Read the model definition and answer for the solid it produces. Units are mm, in the model's axes. A direction names the side the tool comes from. Coordinates: 2 decimals unless noted, no trailing zeros. Loops run counter-clockwise (first coordinate to the right, second up) from the corner with the lowest first, then second, coordinate; pieces in that order, holes last.
Q1. Section C-C (y = 0.3) is taken. Count the separate pieces of the cut face and the enclosed holes in it, then the cut area to 3 significant figures.
Q2. Flat-ended cylindrical pins translate along their axes: P1, Ø0.8, axis at y = 1, z = 2.5, coming from the +X side; P2, Ø0.5, axis at x = 29.5, y = 1, coming from the +Z side; P3, Ø0.8, axis at y = 0.5, z = -3.5, coming from the -X side. Find the tip coordinate at first contact, or state that the pin passes through.
Q3. The mould has two halves that part along X. Classify faces 6 (the face through (7.913, 0.838, 11.535)), 7 (the face through (36.823, 0.838, -16.446)), 8 (the face through (27.461, 0.838, -15.786)), 9 (the face through (1, 1.7, 0)): pulls with the +X half, pulls with the -X half, needs draft (parallel to the pull), parting line crosses it, or undercut.
Q4. Straight lines are drawn through the part: line 1 (X direction, y = 0.6, z = 15) (3 decimals); line 2 (X direction, y = 1.25, z = -18); line 3 (Z direction, x = 33, y = 0.3). For each, find the intervals that lie inside material, in ascending order.
Q5. Which of the six approach directions +Z, -Z, +X, -X, +Y, -Y give full straight-line access (tool end or side, diameter ignored) to faces 1 (the face through (37, 1, 0)), 2 (the face through (-32.99, 0.84, 8.85)), 3 (the face through (-19.84, 0.84, -8.9)), 4 (the face through (27.213, 0.838, -21.413)), 5 (the face through (-30, 1, 21))?
Q6. Section B-B (z = 15) is taken. Give the vertices of the cut face in (x, y) (3 decimals).
Q7. Section A-A (z = 0) is taken. Give the vertices of the cut face in (x, y) (3 decimals), then the cut area to 3 significant figures.
from build123d import *

# Parameters (mm, degrees)
SKETCH1_R           = 6
SKETCH1_R_2         = 3.625
BOSS_EXTRUDE1_DEPTH = 1.7
CUT_EXTRUDE1_REACH  = 46.687
SKETCH2_W           = 13.125
SKETCH2_H           = 18.5
FILLET1_R           = 3
FILLET2_R           = 2


with BuildPart() as part:
    # Sketch1 → Boss-Extrude1 (new body)
    # profile 1 of 7: a face of its own
    with BuildSketch(Plane(origin=(0, 0, 0), x_dir=(1, 0, 0), z_dir=(0, 1, 0))):
        with BuildLine():
            Line((24.690598923, 25), (-24.690598923, 25))
            Line((-24.690598923, 25), (-27, 21))
            Line((-27, 21), (-31, 21))
            ThreePointArc((-31, 21), (-26.757359313, 19.242640687), (-25, 15))
            ThreePointArc((-25, 15), (-27.325765386, 10.25658351), (-32.5, 9.190524981))
            Line((-32.5, 9.190524981), (-32.5, 5.809475019))
            ThreePointArc((-32.5, 5.809475019), (-27.325765386, 4.74341649), (-25, 0))
            ThreePointArc((-25, 0), (-27.325765386, -4.74341649), (-32.5, -5.809475019))
            Line((-32.5, -5.809475019), (-32.5, -9.190524981))
            ThreePointArc((-32.5, -9.190524981), (-27.325765386, -10.25658351), (-25, -15))
            ThreePointArc((-25, -15), (-26.757359313, -19.242640687), (-31, -21))
            Line((-31, -21), (-27, -21))
            Line((-27, -21), (-24.690598923, -25))
            Line((-24.690598923, -25), (24.690598923, -25))
            Line((24.690598923, -25), (27, -21))
            Line((27, -21), (31, -21))
            ThreePointArc((31, -21), (25.047821822, -14.243974245), (32.5, -9.190524981))
            Line((32.5, -9.190524981), (32.5, -5.809475019))
            ThreePointArc((32.5, -5.809475019), (25, 0), (32.5, 5.809475019))
            Line((32.5, 5.809475019), (32.5, 9.190524981))
            ThreePointArc((32.5, 9.190524981), (25.047821822, 14.243974245), (31, 21))
            Line((31, 21), (27, 21))
            Line((27, 21), (24.690598923, 25))
        make_face()
    # profile 2 of 7: a face of its own
    with BuildSketch(Plane(origin=(0, 0, 0), x_dir=(1, 0, 0), z_dir=(0, 1, 0))):
        with Locations((-31, 15)):
            Circle(SKETCH1_R)
        with Locations(Location((-31, 15, 0), (0, 0, 270))):
            Circle(SKETCH1_R_2, mode=Mode.SUBTRACT)
    # profile 3 of 7: a face of its own
    with BuildSketch(Plane(origin=(0, 0, 0), x_dir=(1, 0, 0), z_dir=(0, 1, 0))):
        with Locations((-31, 0)):
            Circle(SKETCH1_R)
        with Locations(Location((-31, 0, 0), (0, 0, 270))):
            Circle(SKETCH1_R_2, mode=Mode.SUBTRACT)
    # profile 4 of 7: a face of its own
    with BuildSketch(Plane(origin=(0, 0, 0), x_dir=(1, 0, 0), z_dir=(0, 1, 0))):
        with Locations((-31, -15)):
            Circle(SKETCH1_R)
        with Locations(Location((-31, -15, 0), (0, 0, 270))):
            Circle(SKETCH1_R_2, mode=Mode.SUBTRACT)
    # profile 5 of 7: a face of its own
    with BuildSketch(Plane(origin=(0, 0, 0), x_dir=(1, 0, 0), z_dir=(0, 1, 0))):
        with Locations((31, -15)):
            Circle(SKETCH1_R)
        with Locations(Location((31, -15, 0), (0, 0, 270))):
            Circle(SKETCH1_R_2, mode=Mode.SUBTRACT)
    # profile 6 of 7: a face of its own
    with BuildSketch(Plane(origin=(0, 0, 0), x_dir=(1, 0, 0), z_dir=(0, 1, 0))):
        with Locations((31, 0)):
            Circle(SKETCH1_R)
        with Locations(Location((31, 0, 0), (0, 0, 270))):
            Circle(SKETCH1_R_2, mode=Mode.SUBTRACT)
    # profile 7 of 7: a face of its own
    with BuildSketch(Plane(origin=(0, 0, 0), x_dir=(1, 0, 0), z_dir=(0, 1, 0))):
        with Locations((31, 15)):
            Circle(SKETCH1_R)
        with Locations(Location((31, 15, 0), (0, 0, 270))):
            Circle(SKETCH1_R_2, mode=Mode.SUBTRACT)
    extrude(amount=BOSS_EXTRUDE1_DEPTH)

    # Sketch2 → Cut-Extrude1 (cut, up to next)
    with BuildSketch(Plane(origin=(0, 1.7, 0), x_dir=(1, 0, 0), z_dir=(0, 1, 0)), mode=Mode.PRIVATE) as cut_extrude1_sk1:
        with Locations((-13.6875, 0)):
            Rectangle(SKETCH2_W, SKETCH2_H)
    cut_extrude1_tool1 = extrude(cut_extrude1_sk1.sketch, amount=-CUT_EXTRUDE1_REACH, mode=Mode.PRIVATE) & part.part
    # Sketch2 → Cut-Extrude1 (cut, up to next)
    with BuildSketch(Plane(origin=(0, 1.7, 0), x_dir=(1, 0, 0), z_dir=(0, 1, 0)), mode=Mode.PRIVATE) as cut_extrude1_sk2:
        Polygon((-7.125, 9.25), (-7.125, 12.5), (-20.25, 9.25), align=None)
    cut_extrude1_tool2 = extrude(cut_extrude1_sk2.sketch, amount=-CUT_EXTRUDE1_REACH, mode=Mode.PRIVATE) & part.part
    # Sketch2 → Cut-Extrude1 (cut, up to next)
    with BuildSketch(Plane(origin=(0, 1.7, 0), x_dir=(1, 0, 0), z_dir=(0, 1, 0)), mode=Mode.PRIVATE) as cut_extrude1_sk3:
        Polygon((-7.125, -12.5), (-7.125, -9.25), (-20.25, -9.25), align=None)
    cut_extrude1_tool3 = extrude(cut_extrude1_sk3.sketch, amount=-CUT_EXTRUDE1_REACH, mode=Mode.PRIVATE) & part.part
    # Sketch2 → Cut-Extrude1 (cut, up to next)
    with BuildSketch(Plane(origin=(0, 1.7, 0), x_dir=(1, 0, 0), z_dir=(0, 1, 0)), mode=Mode.PRIVATE) as cut_extrude1_sk4:
        Polygon((7.125, -12.5), (20.25, -9.25), (7.125, -9.25), align=None)
    cut_extrude1_tool4 = extrude(cut_extrude1_sk4.sketch, amount=-CUT_EXTRUDE1_REACH, mode=Mode.PRIVATE) & part.part
    # Sketch2 → Cut-Extrude1 (cut, up to next)
    with BuildSketch(Plane(origin=(0, 1.7, 0), x_dir=(1, 0, 0), z_dir=(0, 1, 0)), mode=Mode.PRIVATE) as cut_extrude1_sk5:
        with Locations((13.6875, 0)):
            Rectangle(SKETCH2_W, SKETCH2_H)
    cut_extrude1_tool5 = extrude(cut_extrude1_sk5.sketch, amount=-CUT_EXTRUDE1_REACH, mode=Mode.PRIVATE) & part.part
    # Sketch2 → Cut-Extrude1 (cut, up to next)
    with BuildSketch(Plane(origin=(0, 1.7, 0), x_dir=(1, 0, 0), z_dir=(0, 1, 0)), mode=Mode.PRIVATE) as cut_extrude1_sk6:
        Polygon((20.25, 9.25), (7.125, 12.5), (7.125, 9.25), align=None)
    cut_extrude1_tool6 = extrude(cut_extrude1_sk6.sketch, amount=-CUT_EXTRUDE1_REACH, mode=Mode.PRIVATE) & part.part
    add(cut_extrude1_tool1.solids().sort_by_distance((-13.6875, 1.7, 0))[0], mode=Mode.SUBTRACT)
    add(cut_extrude1_tool2.solids().sort_by_distance((-11.5, 1.7, -10.333333))[0], mode=Mode.SUBTRACT)
    add(cut_extrude1_tool3.solids().sort_by_distance((-11.5, 1.7, 10.333333))[0], mode=Mode.SUBTRACT)
    add(cut_extrude1_tool4.solids().sort_by_distance((11.5, 1.7, 10.333333))[0], mode=Mode.SUBTRACT)
    add(cut_extrude1_tool5.solids().sort_by_distance((13.6875, 1.7, 0))[0], mode=Mode.SUBTRACT)
    add(cut_extrude1_tool6.solids().sort_by_distance((11.5, 1.7, -10.333333))[0], mode=Mode.SUBTRACT)

    # Fillet1
    # the kernel refuses this fillet: 3 mm, written as the material it adds along each edge
    with BuildSketch(Plane(origin=(32.5, 0, 9.190524981), x_dir=(0, 0, -1), z_dir=(0, 1, 0)), Plane(origin=(32.5, 0, -5.809475019), x_dir=(0, 0, -1), z_dir=(0, 1, 0))) as fillet1_piece_1:
        with BuildLine():
            CenterArc((1.984753615, -3), FILLET1_R, 90, 60)
            ThreePointArc((-0.613322597, -1.5), (-0.255786259, -0.770801874), (0, 0))
            Line((0, 0), (1.984753615, 0))
        make_face()
    extrude(amount=1.7)
    with BuildSketch(Plane(origin=(32.5, 0, 5.809475019), x_dir=(0.9256147934109572, 0, -0.3784669790335627), z_dir=(0, 1, 0)), Plane(origin=(32.5, 0, -9.190524981), x_dir=(0.9256147934109562, 0, -0.378466979033565), z_dir=(0, 1, 0))) as fillet1_piece_2:
        with BuildLine():
            CenterArc((2.025680676, -2.972518244), FILLET1_R, 97.761243907, 60)
            Line((-0.751163705, -1.837117307), (0, 0))
            ThreePointArc((0, 0), (0.81027227, -0.054963512), (1.62054454, 0))
        make_face()
    extrude(amount=1.7)
    with BuildSketch(Plane(origin=(-32.5, 0, 9.190524981), x_dir=(0, 0, -1), z_dir=(0, 1, 0)), Plane(origin=(-32.5, 0, -5.809475019), x_dir=(0, 0, -1), z_dir=(0, 1, 0))) as fillet1_piece_3:
        with BuildLine():
            CenterArc((1.984753615, 3), FILLET1_R, 210, 60)
            ThreePointArc((-0.613322597, 1.5), (-0.255786259, 0.770801874), (0, 0))
            Line((0, 0), (1.984753615, 0))
        make_face()
    extrude(amount=1.7)
    with BuildSketch(Plane(origin=(-32.5, 0, 5.809475019), x_dir=(-0.9256147934109573, 0, -0.3784669790335622), z_dir=(0, 1, 0)), Plane(origin=(-32.5, 0, -9.190524981), x_dir=(-0.9256147934109568, 0, -0.37846697903356347), z_dir=(0, 1, 0))) as fillet1_piece_4:
        with BuildLine():
            CenterArc((2.025680676, 2.972518244), FILLET1_R, 202.238756093, 60)
            Line((-0.751163705, 1.837117307), (0, 0))
            ThreePointArc((0, 0), (0.81027227, 0.054963512), (1.62054454, 0))
        make_face()
    extrude(amount=1.7)
    with BuildSketch(Plane(origin=(-27, 0, 21), x_dir=(0.49999999999999767, 0, 0.8660254037844399), z_dir=(0, 1, 0)), Plane(origin=(27, 0, 21), x_dir=(1, 0, 0), z_dir=(0, 1, 0))) as fillet1_piece_5:
        with BuildLine():
            CenterArc((FILLET1_R * 0.57735026919, -FILLET1_R), FILLET1_R, 90, 60)
            Line((-FILLET1_R * 0.288675134595, -FILLET1_R * 0.5), (0, 0))
            Line((0, 0), (FILLET1_R * 0.57735026919, 0))
        make_face()
    extrude(amount=1.7)
    with BuildSketch(Plane(origin=(27, 0, -21), x_dir=(1, 0, 0), z_dir=(0, 1, 0)), Plane(origin=(-27, 0, -21), x_dir=(0.49999999999999767, 0, -0.8660254037844399), z_dir=(0, 1, 0))) as fillet1_piece_6:
        with BuildLine():
            CenterArc((FILLET1_R * 0.57735026919, FILLET1_R), FILLET1_R, 210, 60)
            Line((-FILLET1_R * 0.288675134595, FILLET1_R * 0.5), (0, 0))
            Line((0, 0), (FILLET1_R * 0.57735026919, 0))
        make_face()
    extrude(amount=1.7)
    # the kernel refuses this fillet: 3 mm, written as the material it takes off along each edge
    with BuildSketch(Plane(origin=(-24.690598923, -4.330127019, 25), x_dir=(1, 0, 0), z_dir=(0, 1, 0)), Plane(origin=(24.690598923, -4.330127019, 25), x_dir=(0.49999999999999767, 0, -0.8660254037844399), z_dir=(0, 1, 0))) as fillet1_2_piece_1:
        with BuildLine():
            CenterArc((FILLET1_R * 0.57735026919, FILLET1_R), FILLET1_R, 210, 60)
            Line((-FILLET1_R * 0.288675134595, FILLET1_R * 0.5), (0, 0))
            Line((0, 0), (FILLET1_R * 0.57735026919, 0))
        make_face()
    extrude(amount=10.360254038, mode=Mode.SUBTRACT)
    with BuildSketch(Plane(origin=(24.690598923, -4.330127019, -25), x_dir=(0.49999999999999767, 0, 0.8660254037844399), z_dir=(0, 1, 0)), Plane(origin=(-24.690598923, -4.330127019, -25), x_dir=(1, 0, 0), z_dir=(0, 1, 0))) as fillet1_2_piece_2:
        with BuildLine():
            CenterArc((FILLET1_R * 0.57735026919, -FILLET1_R), FILLET1_R, 90, 60)
            Line((-FILLET1_R * 0.288675134595, -FILLET1_R * 0.5), (0, 0))
            Line((0, 0), (FILLET1_R * 0.57735026919, 0))
        make_face()
    extrude(amount=10.360254038, mode=Mode.SUBTRACT)

    # Fillet2
    fillet2_edges = [part.edges().sort_by_distance(p)[0] for p in [
        (-20.25, 0.85, 9.25),
        (-20.25, 0.85, -9.25),
        (-7.125, 0.85, -12.5),
        (-7.125, 0.85, 12.5),
        (20.25, 0.85, 9.25),
        (7.125, 0.85, 12.5),
        (7.125, 0.85, -12.5),
        (20.25, 0.85, -9.25),
    ]]
    fillet(fillet2_edges, radius=FILLET2_R)


solid = part.part
Numbers:
1. separate pieces: 1
1. enclosed holes: 8
1. area: 2,570 mm2
2. P1: stops at x = 36.62
2. P2: stops at z = 21
2. P3: stops at x = -36.14
3. face 6: undercut
3. face 7: pulls with the +X half
3. face 8: undercut
3. face 9: needs draft
4. line 1: x = -37 to -34.625, -27.375 to 27.375, 34.625 to 37
4. line 2: x = -36.2 to -33.03, -28.97 to 28.97, 33.03 to 36.2
4. line 3: z = -20.66 to -18.02, -11.98 to -8.86, -6.14 to -3.02, 3.02 to 6.14, 8.86 to 11.98, 18.02 to 20.66
5. face 1: +X, +Y, -Y
5. face 2: -X, +Y, -Y
5. face 3: +Y, -Y
5. face 4: -Z, +X, +Y, -Y
5. face 5: +Z, -X, +Y, -Y
6. outline: (-37, 0) - (-34.625, 0) - (-34.625, 1.7) - (-37, 1.7) - close; (-27.375, 0) - (27.375, 0) - (27.375, 1.7) - (-27.375, 1.7) - close; (34.625, 0) - (37, 0) - (37, 1.7) - (34.625, 1.7) - close
7. outline: (-37, 0) - (-34.625, 0) - (-34.625, 1.7) - (-37, 1.7) - close; (-27.375, 0) - (-20.25, 0) - (-20.25, 1.7) - (-27.375, 1.7) - close; (-7.125, 0) - (7.125, 0) - (7.125, 1.7) - (-7.125, 1.7) - close; (20.25, 0) - (27.375, 0) - (27.375, 1.7) - (20.25, 1.7) - close; (34.625, 0) - (37, 0) - (37, 1.7) - (34.625, 1.7) - close
7. area: 56.5 mm2
